Build history of the part. All positions in model axes, mm. A direction names the side the tool comes from. Round coordinates to 2 decimals unless told otherwise and drop trailing zeros. Write each loop counter-clockwise with the first axis right and the second up, starting at its lowest first coordinate (ties: lowest second). Pieces come first, ordered by that corner, then holes.
from build123d import *

# Parameters (mm, degrees)
EXTRUDE_1_OUTLINE_R = 2
EXTRUDE_1_DEPTH     = 5.1
SKETCH_4_2_R        = 2
CUT_EXTRUDE_1_DEPTH = 2.1
SKETCH_5_R          = 0.75
CUT_EXTRUDE_2_DEPTH = 48.355992497
FILLET_1_R          = 0.5
FILLET_2_R          = 3


with BuildPart() as part:
    # 凸台-拉伸1: read off the stored shape, not the designer's step
    # 凸台-拉伸1 outline → 凸台-拉伸1 (new body)
    with BuildSketch(Plane(origin=(15.11890087, 0, 4.548317805), x_dir=(-0.8371072123201975, 0, -0.5470388606685158), z_dir=(0.5470388606685158, 0, -0.8371072123201975))):
        with BuildLine():
            ThreePointArc((-11.855752449, -22), (-15.855752449, -26), (-11.855752449, -30))
            ThreePointArc((-11.855752449, -30), (2.877521805, -28.097510014), (16.644247551, -22.514849302))
            Line((16.644247551, -22.514849302), (16.644247551, -21))
            Line((16.644247551, -21), (19.644247551, -21))
            Line((19.644247551, -21), (19.644247551, -25))
            Line((19.644247551, -25), (31.644247551, -25))
            Line((31.644247551, -25), (31.644247551, -21))
            Line((31.644247551, -21), (34.644247551, -21))
            Line((34.644247551, -21), (34.644247551, -6.666266023))
            ThreePointArc((34.644247551, -6.666266023), (43.194224844, 9.738017632), (46.144247551, 28))
            Line((46.144247551, 28), (46.144247551, 33.2))
            Line((46.144247551, 33.2), (38.144247551, 33.2))
            Line((38.144247551, 33.2), (38.144247551, 28))
            ThreePointArc((38.144247551, 28), (23.49958661, -7.355339059), (-11.855752449, -22))
        make_face()
        with Locations((-11.855752449, -26)):
            Circle(EXTRUDE_1_OUTLINE_R, mode=Mode.SUBTRACT)
        with Locations((0.160377984, -24.646107258)):
            Circle(EXTRUDE_1_OUTLINE_R, mode=Mode.SUBTRACT)
        with Locations((11.573969463, -20.652318867)):
            Circle(EXTRUDE_1_OUTLINE_R, mode=Mode.SUBTRACT)
        with Locations((21.812696851, -14.218900053)):
            Circle(EXTRUDE_1_OUTLINE_R, mode=Mode.SUBTRACT)
        with Locations((30.363147604, -5.6684493)):
            Circle(EXTRUDE_1_OUTLINE_R, mode=Mode.SUBTRACT)
        with Locations((36.796566418, 4.570278088)):
            Circle(EXTRUDE_1_OUTLINE_R, mode=Mode.SUBTRACT)
        with Locations((40.790354809, 15.983869566)):
            Circle(EXTRUDE_1_OUTLINE_R, mode=Mode.SUBTRACT)
        with Locations((42.144247551, 28)):
            Circle(EXTRUDE_1_OUTLINE_R, mode=Mode.SUBTRACT)
    extrude(amount=EXTRUDE_1_DEPTH)

    # 草图4<2> → 切除-拉伸1 (cut)
    with BuildSketch(Plane(origin=(15.11890087, 0, 4.548317805), x_dir=(-0.8371072123201975, 0, -0.5470388606685158), z_dir=(0.5470388606685158, 0, -0.8371072123201975))):
        with BuildLine():
            Line((19.644247551, -21), (19.644247551, -25))
            Line((19.644247551, -25), (31.644247551, -25))
            Line((31.644247551, -25), (31.644247551, -21))
            Line((31.644247551, -21), (34.644247551, -21))
            Line((34.644247551, -21), (34.644247551, -6.666266023))
            ThreePointArc((34.644247551, -6.666266023), (43.194224844, 9.738017632), (46.144247551, 28))
            Line((46.144247551, 28), (46.144247551, 33.2))
            Line((46.144247551, 33.2), (38.144247551, 33.2))
            Line((38.144247551, 33.2), (38.144247551, 28))
            ThreePointArc((38.144247551, 28), (23.49958661, -7.355339059), (-11.855752449, -22))
            ThreePointArc((-11.855752449, -22), (-15.855752449, -26), (-11.855752449, -30))
            ThreePointArc((-11.855752449, -30), (2.877521805, -28.097510014), (16.644247551, -22.514849302))
            Line((16.644247551, -22.514849302), (16.644247551, -21))
            Line((16.644247551, -21), (19.644247551, -21))
        make_face()
        with Locations((42.144247551, 28)):
            Circle(SKETCH_4_2_R, mode=Mode.SUBTRACT)
        with Locations((40.790354809, 15.983869566)):
            Circle(SKETCH_4_2_R, mode=Mode.SUBTRACT)
        with Locations((36.796566418, 4.570278088)):
            Circle(SKETCH_4_2_R, mode=Mode.SUBTRACT)
        with Locations((30.363147604, -5.6684493)):
            Circle(SKETCH_4_2_R, mode=Mode.SUBTRACT)
        with Locations((21.812696851, -14.218900053)):
            Circle(SKETCH_4_2_R, mode=Mode.SUBTRACT)
        with Locations((11.573969463, -20.652318867)):
            Circle(SKETCH_4_2_R, mode=Mode.SUBTRACT)
        with Locations((0.160377984, -24.646107258)):
            Circle(SKETCH_4_2_R, mode=Mode.SUBTRACT)
        with Locations((-11.855752449, -26)):
            Circle(SKETCH_4_2_R, mode=Mode.SUBTRACT)
    extrude(amount=CUT_EXTRUDE_1_DEPTH, mode=Mode.SUBTRACT)

    # 草图5 → 切除-拉伸2 (cut, through all)
    with BuildSketch(Plane(origin=(5.23144021, 0, -8.005420904), x_dir=(-0.8371072123201976, 0, -0.5470388606685158), z_dir=(0.5470388606685158, 0, -0.8371072123201976))):
        with Locations((3.75, -21)):
            Circle(SKETCH_5_R)
        with Locations((16.5, -21)):
            Circle(SKETCH_5_R)
        with Locations((1.5, -21)):
            Circle(SKETCH_5_R)
    extrude(amount=-CUT_EXTRUDE_2_DEPTH, mode=Mode.SUBTRACT)

    # 圆角1
    fillet_1_edges = [part.edges().sort_by_distance(p)[0] for p in [
        (-10.029217494, -21, -16.186180432),
        (3.1552211, -22.514849302, -7.570318376),
    ]]
    fillet(fillet_1_edges, radius=FILLET_1_R)

    # 圆角2
    fillet_2_edges = [part.edges().sort_by_distance(p)[0] for p in [
        (-11.912708722, -6.666266023, -17.417017868),
    ]]
    fillet(fillet_2_edges, radius=FILLET_2_R)


solid = part.part
1) Mould opens along Z. For faces 1 (the flat face through (-11, -21, -17)), 2 (the flat face through (-14.854, 30.636, -19.314)), 3 (the cylindrical face through (3.596, -20.452, -7.308)) say: released by +Z, released by -Z, zero draft, split by the parting line, or undercut.
Results:
face 1: zero draft
face 2: released by +Z
face 3: undercut
2) Which spindle directions (+Z, -Z, +X, -X, +Y, -Y) get a long thin tool onto all of the face, cutting with end or side? Do faces 4 (the flat face through (0.63, -22.97, -9.19)), 5 (the cylindrical face through (-8.123, -3.685, -14.915)), 6 (the flat face through (-11.924, -14.417, -17.399)), 7 (the flat face through (3.14, -21.99, -7.55)), 8 (the flat face through (-3.98, -9.96, -10.44)). Say none if no direction does.
Results:
face 4: +Z, -Y
face 5: none
face 6: -Z, -X, -Y
face 7: -Z, -Y
face 8: +Z, -X, +Y, -Y
3) Slice it at A-A (y = 8.5). Write the cut outline in (x, z).
Results:
outline: (-19.53, -20.61) - (-17.89, -23.12) - (-10.71, -18.42) - (-12.35, -15.91) - close
4) Pin check, flat tips, straight feed: pin 1 Ø1.8 at (x, z) = (2.5, -7.5) entering from -Y; pin 2 Ø2.5 at (x, z) = (-5, -12.5) entering from -Y; pin 3 Ø2.5 at (x, z) = (-11.5, -17.5) entering from -Y. Stop position of each tip, or through.
Results:
pin 1: stops at y = -22.73
pin 2: stops at y = -25
pin 3: stops at y = -21
5) Wall check: L1, parallel to Y at x = 26.5, z = 6; L2, parallel to X at y = -14, z = -18.5 (3 decimals); L3, parallel to X at y = 2.5, z = -21.5. Give the ranges that are in metal, low to high.
Results:
L1: y = -29.98 to -27.28, -24.72 to -21.98
L2: x = -11.205 to -10.828
L3: x = -15.93 to -15.42
